The listing builds one solid part. Answer for the finished solid, in the listing's coordinates (mm). Give positions to 0.01 mm unless a question says otherwise; leave off trailing zeros. Loops run counter-clockwise (first coordinate to the right, second up) from the corner with the lowest first, then second, coordinate; pieces in that order, holes last. Notation, with made-up numbers: (-21, -25) - (26, -25) arc R22 ccw to (26, 9) - close; hole circle Ø11 at (-14, 48). An arc over 180 degrees is marked (long way). One line per item, written item: value. Start each with the question number.
from build123d import *

# Parameters (mm, degrees)
SKETCH1_R           = 6.45
SKETCH1_R_2         = 2.5
SKETCH1_W           = 20.5
SKETCH1_H           = 40.7
BOSS_EXTRUDE1_DEPTH = 3.1
SKETCH2_W           = 20.093106281
SKETCH2_H           = 3.1
SKETCH2_W_2         = 20
CUT_EXTRUDE1_DEPTH  = 4.1


with BuildPart() as part:
    # Sketch1 → Boss-Extrude1 (new body)
    with BuildSketch(Plane.XY):
        with BuildLine():
            Line((-20, 0), (-20, 224.85))
            Line((-20, 224.85), (20, 224.85))
            Line((20, 224.85), (20, 0))
            ThreePointArc((20, 0), (0, -20), (-20, 0))
        make_face()
        Circle(SKETCH1_R, mode=Mode.SUBTRACT)
        with Locations((5, 145.85)):
            Circle(SKETCH1_R_2, mode=Mode.SUBTRACT)
        with Locations((-5, 145.85)):
            Circle(SKETCH1_R_2, mode=Mode.SUBTRACT)
        with Locations((-5, 194.85)):
            Circle(SKETCH1_R_2, mode=Mode.SUBTRACT)
        with Locations((5, 194.85)):
            Circle(SKETCH1_R_2, mode=Mode.SUBTRACT)
        with Locations((0, 170.35)):
            Rectangle(SKETCH1_W, SKETCH1_H, mode=Mode.SUBTRACT)
    extrude(amount=BOSS_EXTRUDE1_DEPTH)

    # Sketch2 → Cut-Extrude1 (cut, through all)
    with BuildSketch(Plane.XY.offset(3.1)):
        with Locations((10.046553141, 223.3)):
            Rectangle(SKETCH2_W, SKETCH2_H)
        with Locations((10, 133.45)):
            Rectangle(SKETCH2_W_2, SKETCH2_H)
    extrude(amount=-CUT_EXTRUDE1_DEPTH, mode=Mode.SUBTRACT)


solid = part.part
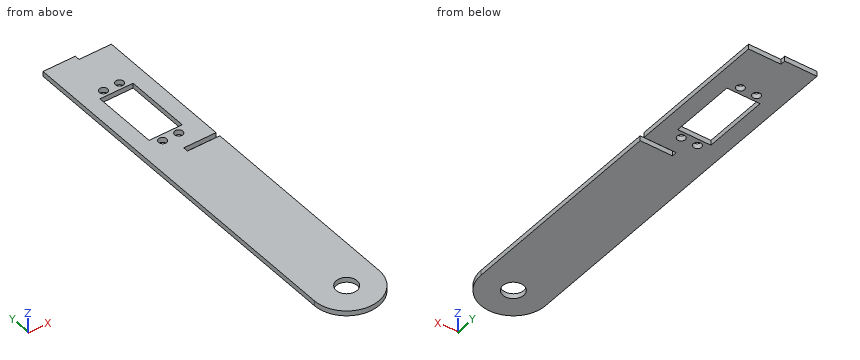
1. A cutting plane is placed at A-A (y = 194.85). Determine the outline of the cut face in (x, z).
2. A cutting plane is placed at B-B (z = 2.6). Determine the outline of the cut face in (x, y), plus the area to 3 significant figures.
3. Find the intervals of material crossed by L1, parallel to X at y = 145.85, z = 1.2; L2, parallel to X at y = 175, z = 2.4; L3, parallel to Y at x = -5, z = 0.85, in increasing order. Write a range as [from, to].
4. Flat-ended cylindrical pins translate along their axes: pin 1 (1.6 mm diameter, centred on x = 10.5, z = 2, fed in from -Y); pin 2 (5 mm diameter, centred on x = -15, y = 181.5, fed in from -Z); pin 3 (1.6 mm diameter, centred on x = 5, z = 1, fed in from +Y). Find the tip coordinate at first contact, or state that the pin passes through.
Results below:
1. outline: (-20, 0) - (-7.5, 0) - (-7.5, 3.1) - (-20, 3.1) - close; (-2.5, 0) - (2.5, 0) - (2.5, 3.1) - (-2.5, 3.1) - close; (7.5, 0) - (20, 0) - (20, 3.1) - (7.5, 3.1) - close
2. outline: (-20, 0) arc R20 ccw to (20, 0) - (20, 131.9) - (0, 131.9) - (0, 135) - (20, 135) - (20, 221.75) - (0, 221.75) - (0, 224.85) - (-20, 224.85) - close; hole (-10.25, 150) - (10.25, 150) - (10.25, 190.7) - (-10.25, 190.7) - close; hole circle Ø5 at (-5, 145.85); hole circle Ø5 at (-5, 194.85); hole circle Ø12.9 at (0, 0); hole circle Ø5 at (5, 145.85); hole circle Ø5 at (5, 194.85)
2. area: 8,450 mm^2
3. L1: x = [-20, -7.5], [-2.5, 2.5], [7.5, 20]
3. L2: x = [-20, -10.25], [10.25, 20]
3. L3: y = [-19.36, -4.07], [4.07, 143.35], [148.35, 150], [190.7, 192.35], [197.35, 224.85]
4. pin 1: stops at y = -17.49
4. pin 2: stops at z = 0
4. pin 3: stops at y = 221.75
